Design review of the part shown in the three views and the two pictorial views. Dimensions are in mm from the part's minimum x, y and z. A direction names the side the tool comes from. Round coordinates to 2 decimals unless told otherwise and drop trailing zeros. Write each loop counter-clockwise with the first axis right and the second up, starting at its lowest first coordinate (ties: lowest second). Pieces come first, ordered by that corner, then holes. Notation, with made-up numbers: (60, 14.5) - (70, 14.5) arc R21 cw to (70, 42.5) - close; hole circle Ø4 at (79.25, 31). An arc over 180 degrees is marked (long way). Use one line per item in the form item = value.
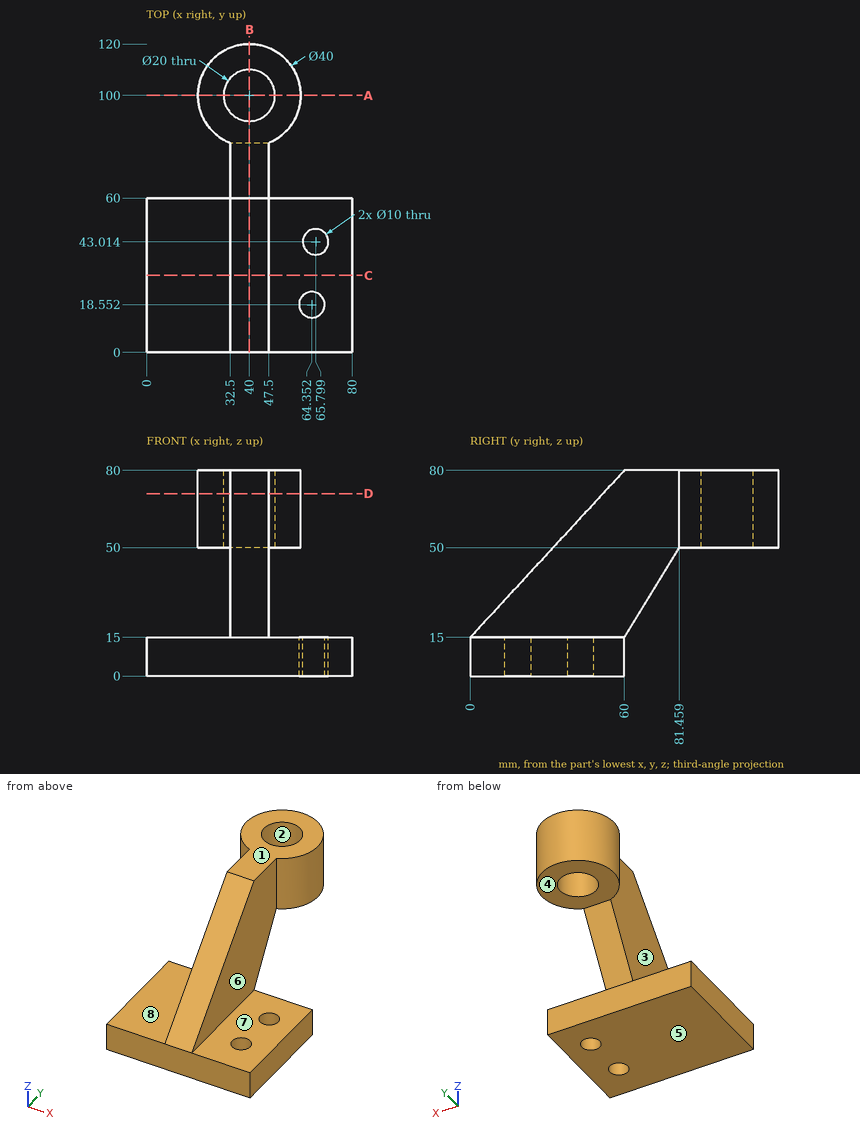
(1) Add section D-D on z = 71. Write out the cut boundary in (x, y).
Geometry results:
outline = (32.5, 51.69) - (47.5, 51.69) - (47.5, 81.46) arc R20 ccw (long way) to (32.5, 81.46) - close; hole circle Ø20 at (40, 100)
(2) Machinability: for the marked faces 4, 5, 6, 7 and 8, which of the approach directions +Z, -Z, +X, -X, +Y, -Y give a long, thin tool a straight path to every point of the face, cutting with its end or side? Answer none if there is none.
Geometry results:
face_4 = -Z, +X, -X, +Y
face_5 = -Z, +X, -X, +Y, -Y
face_6 = +Z, +X, -Y
face_7 = +Z, +X, +Y, -Y
face_8 = +Z, -X, +Y, -Y
(3) Add section A-A on y = 100. Write out the cut boundary in (x, z), then the cut area to 3 significant figures.
Geometry results:
outline = (20, 50) - (30, 50) - (30, 80) - (20, 80) - close; (50, 50) - (60, 50) - (60, 80) - (50, 80) - close
area = 600 mm2
(4) Add section C-C on y = 30. Write out the cut boundary in (x, z).
Geometry results:
outline = (0, 0) - (80, 0) - (80, 15) - (47.5, 15) - (47.5, 47.5) - (32.5, 47.5) - (32.5, 15) - (0, 15) - close
(5) The part is to be moulded in two halves that separate along X. For the marked faces 1, 2 and 3, say which applies: +X half, -X half, draft (parallel to the pull), parting line (faces both ways), or undercut.
Geometry results:
face_1 = draft
face_2 = undercut
face_3 = -X half
(6) Insertion check: P1, Ø16, axis at x = 14, y = 21.5, coming from the +Z side; P2, Ø2, axis at x = 34, y = 72.5, coming from the -Z side (1 decimal); P3, Ø9, axis at x = 64.35, y = 18.55, coming from the +Z side; P4, Ø12, axis at x = 43.5, z = 17, coming from the +Y side (1 decimal). Each pin has a flat end and moves straight along its axis. Give the tip position at first contact, or say it passes through.
Geometry results:
P1 = 15
P2 = 33.8
P3 = through
P4 = 64.9
(7) To check wall thickness, follow L1, parallel to X at y = 100, z = 73; L2, parallel to Y at x = 39.5, z = 13; L3, parallel to Z at x = 19.5, y = 13.5. State the ranges of each line that lie inside material, in increasing order.
Geometry results:
L1 = 20 to 30, 50 to 60
L2 = 0 to 60
L3 = 0 to 15
(8) Add section B-B on x = 40. Write out the cut boundary in (y, z).
Geometry results:
outline = (0, 0) - (60, 0) - (60, 15) - (81.46, 50) - (90, 50) - (90, 80) - (60, 80) - (0, 15) - close; (110, 50) - (120, 50) - (120, 80) - (110, 80) - close
